Geometry check sheet. Reference: the model listing, model coordinates, mm. Give positions to 0.01 mm unless a question says otherwise; leave off trailing zeros. Loops run counter-clockwise (first coordinate to the right, second up) from the corner with the lowest first, then second, coordinate; pieces in that order, holes last.
1. Material ranges on L1, parallel to Z at x = -4, y = 5; L2, parallel to Z at x = -6, y = 1.5; L3, parallel to Z at x = 9.5, y = 14.5, recorded low to high.
2. Cross-section at A-A, the plane z = -73. Record the cut outline in (x, y), plus the area to 3 significant figures.
3. Cross-section at B-B, the plane y = 12. State how many separate pieces and enclosed holes the cut face has, plus the area to 3 significant figures.
4. Cross-section at C-C, the plane z = -225. Record the cut outline in (x, y).
5. Go/stop test with flat-tipped pins: pin 1 Ø7.5 at (y, z) = (8, -90) entering from +X; pin 2 Ø23.5 at (x, z) = (0, -250) entering from +Y; pin 3 Ø6.5 at (y, z) = (8, -199) entering from -X; pin 4 Ø5 at (x, y) = (-2.5, 3) entering from -Z. Record where each tip stops, or that it passes through.
from build123d import *

# Parameters (mm, degrees)
SKETCH_1_R          = 5.05
SKETCH_1_R_2        = 13
EXTRUDE_1_DEPTH     = 15
FILLET_1_R          = 3
SKETCH_7_R          = 2.05
CUT_EXTRUDE_4_DEPTH = 277.54113618
SKETCH_8_R          = 13
CUT_EXTRUDE_5_DEPTH = 277.54113618
SKETCH_9_R          = 25
SKETCH_9_R_2        = 13
EXTRUDE_4_DEPTH     = 15
SKETCH_10_R         = 1.5
EXTRUDE_5_DEPTH     = 15
EXTRUDE_START       = -15
SKETCH_14_R         = 13
SKETCH_14_R_2       = 9
EXTRUDE_6_DEPTH     = 15
SKETCH_13_R         = 23.5
SKETCH_13_R_2       = 1.5
CUT_EXTRUDE_6_DEPTH = 25
CUT_EXTRUDE_START   = -15
CUT_EXTRUDE_7_DEPTH = 15
EXTRUDE_9_DEPTH     = 15
CUT_EXTRUDE_8_DEPTH = 30


# Read off the part's stored shape, not the designer's step: 切除-拉伸7
with BuildPart() as part:
    # 草图1 → 凸台-拉伸1 (new body)
    with BuildSketch(Plane(origin=(0, 0, 0), x_dir=(1, 0, 0), z_dir=(0, 1, 0))):
        with BuildLine():
            Line((-17.992942616, -0.504), (-24.990198078, 249.3))
            ThreePointArc((-24.990198078, 249.3), (0, 275), (24.990198078, 249.3))
            Line((24.990198078, 249.3), (17.992942616, -0.504))
            ThreePointArc((17.992942616, -0.504), (0, -18), (-17.992942616, -0.504))
        make_face()
        with Locations(Location((0, 0, 0), (0, 0, 270))):
            Circle(SKETCH_1_R, mode=Mode.SUBTRACT)
        with Locations(Location((0, 250, 0), (0, 0, 270))):
            Circle(SKETCH_1_R_2, mode=Mode.SUBTRACT)
        Polygon((-16.444447487, 158.5), (-17.704941698, 203.5), (11.028871219, 137.174942267), align=None, mode=Mode.SUBTRACT)
        Polygon((15.954255294, 141), (18.475243716, 231), (-12, 219.5), align=None, mode=Mode.SUBTRACT)
    extrude(amount=EXTRUDE_1_DEPTH)

    # 圆角1
    fillet_1_edges = [part.edges().sort_by_distance(p)[0] for p in [
        (-16.444447487, 7.5, -158.5),
        (11.028871219, 7.5, -137.174942267),
        (-17.704941698, 7.5, -203.5),
        (18.475243716, 7.5, -231),
        (-12, 7.5, -219.5),
        (15.954255294, 7.5, -141),
    ]]
    fillet(fillet_1_edges, radius=FILLET_1_R)

    # 草图7 → 切除-拉伸4 (cut, through all)
    with BuildSketch(Plane(origin=(0, 15, 0), x_dir=(1, 0, 0), z_dir=(0, 1, 0))):
        with Locations(Location((15, 15, 0), (0, 0, 270))):
            Circle(SKETCH_7_R)
        with Locations(Location((-15, 15, 0), (0, 0, 270))):
            Circle(SKETCH_7_R)
        with Locations((-15, -15)):
            Circle(SKETCH_7_R)
        with Locations((15, -15)):
            Circle(SKETCH_7_R)
    extrude(amount=-CUT_EXTRUDE_4_DEPTH, mode=Mode.SUBTRACT)

    # 草图8 → 切除-拉伸5 (cut, through all)
    with BuildSketch(Plane(origin=(0, 15, 0), x_dir=(1, 0, 0), z_dir=(0, 1, 0))):
        with Locations(Location((0, 0, 0), (0, 0, 270))):
            Circle(SKETCH_8_R)
    extrude(amount=-CUT_EXTRUDE_5_DEPTH, mode=Mode.SUBTRACT)

    # 草图9 → 凸台-拉伸4 (add)
    with BuildSketch(Plane(origin=(0, 15, 0), x_dir=(1, 0, 0), z_dir=(0, 1, 0))):
        Circle(SKETCH_9_R)
        with Locations(Location((0, 0, 0), (0, 0, 270))):
            Circle(SKETCH_9_R_2, mode=Mode.SUBTRACT)
    extrude(amount=-EXTRUDE_4_DEPTH)

    # 草图10 → 凸台-拉伸5 (add)
    with BuildSketch(Plane(origin=(0, 15, 0), x_dir=(1, 0, 0), z_dir=(0, 1, 0))):
        with BuildLine():
            Line((-39.711049207, 4.799226071), (-40, 0))
            ThreePointArc((-40, 0), (0, -40), (40, 0))
            Line((40, 0), (39.711049207, 4.799226071))
            Line((39.711049207, 4.799226071), (24.990198078, 249.3))
            Line((24.990198078, 249.3), (18.993134598, 35.203136766))
            Line((18.993134598, 35.203136766), (18.478724461, 16.838549294))
            ThreePointArc((18.478724461, 16.838549294), (0, -25), (-18.478724461, 16.838549294))
            Line((-18.478724461, 16.838549294), (-18.993134598, 35.203136766))
            Line((-18.993134598, 35.203136766), (-24.990198078, 249.3))
            Line((-24.990198078, 249.3), (-39.711049207, 4.799226071))
        make_face()
        with Locations(Location((-31.493406412, -20.357194124, 0), (0, 0, 270))):
            Circle(SKETCH_10_R, mode=Mode.SUBTRACT)
        with Locations(Location((-37.210701127, 4.649055992, 0), (0, 0, 270))):
            Circle(SKETCH_10_R, mode=Mode.SUBTRACT)
        with Locations(Location((-25.516695234, 27.479961141, 0), (0, 0, 270))):
            Circle(SKETCH_10_R, mode=Mode.SUBTRACT)
        with Locations(Location((-11.039996826, -35.838086864, 0), (0, 0, 270))):
            Circle(SKETCH_10_R, mode=Mode.SUBTRACT)
        with Locations(Location((14.579149971, -34.549940465, 0), (0, 0, 270))):
            Circle(SKETCH_10_R, mode=Mode.SUBTRACT)
        with Locations(Location((33.376550467, -17.095492942, 0), (0, 0, 270))):
            Circle(SKETCH_10_R, mode=Mode.SUBTRACT)
        with Locations(Location((22.631551157, 29.900884473, 0), (0, 0, 270))):
            Circle(SKETCH_10_R, mode=Mode.SUBTRACT)
        with Locations(Location((36.55669206, 8.358125723, 0), (0, 0, 270))):
            Circle(SKETCH_10_R, mode=Mode.SUBTRACT)
    extrude(amount=-EXTRUDE_5_DEPTH)

    # 草图14 → 凸台-拉伸6 (add)
    with BuildSketch(Plane(origin=(0, 15, 0), x_dir=(1, 0, 0), z_dir=(0, 1, 0)).offset(EXTRUDE_START)):
        with Locations((0, 250)):
            Circle(SKETCH_14_R)
        with Locations(Location((0, 250, 0), (0, 0, 270))):
            Circle(SKETCH_14_R_2, mode=Mode.SUBTRACT)
    extrude(amount=EXTRUDE_6_DEPTH)

    # 草图13 → 切除-拉伸6 (cut)
    with BuildSketch(Plane(origin=(0, 15, 0), x_dir=(1, 0, 0), z_dir=(0, 1, 0))):
        with Locations(Location((0, 0, 0), (0, 0, 270))):
            Circle(SKETCH_13_R)
        with Locations(Location((-1.883144055, 37.452687066, 0), (0, 0, 270))):
            Circle(SKETCH_13_R_2)
    extrude(amount=-CUT_EXTRUDE_6_DEPTH, mode=Mode.SUBTRACT)

    # 切除-拉伸7 outline → 切除-拉伸7 (cut)
    with BuildSketch(Plane(origin=(0, 15, 0), x_dir=(1, 0, 0), z_dir=(0, 1, 0)).offset(CUT_EXTRUDE_START)):
        with BuildLine():
            ThreePointArc((-39.711049207, 4.799226071), (-38.432072473, 11.089445679), (-36.163406358, 17.094093734))
            ThreePointArc((-36.163406358, 17.094093734), (-31.834646693, 28.891099747), (-29.684840552, 41.271965817))
            Line((-29.684840552, 41.271965817), (-18, 250))
            ThreePointArc((-18, 250), (0, 268), (18, 250))
            Line((18, 250), (29.684856444, 41.271998774))
            ThreePointArc((29.684856444, 41.271998774), (31.834654407, 28.891107358), (36.163414547, 17.09407641))
            ThreePointArc((36.163414547, 17.09407641), (38.432075129, 11.089436474), (39.711049207, 4.799226071))
            Line((39.711049207, 4.799226071), (24.990198078, 249.3))
            ThreePointArc((24.990198078, 249.3), (0, 275), (-24.990198078, 249.3))
            Line((-24.990198078, 249.3), (-39.711049207, 4.799226071))
        make_face()
    extrude(amount=CUT_EXTRUDE_7_DEPTH, mode=Mode.SUBTRACT)

    # 草图18 → 凸台-拉伸9 (add)
    with BuildSketch(Plane(origin=(0, 0, 0), x_dir=(-1, 0, 0), z_dir=(0, -1, 0))):
        Polygon((-20.868155543, 131.844626328), (20.706902291, 152.097209515), (16.905995412, 230.591726078), (-18.51031166, 232.603381148), (-19.336560971, 196.02914685), align=None)
    extrude(amount=-EXTRUDE_9_DEPTH)

    # 草图19 → 切除-拉伸8 (cut)
    with BuildSketch(Plane(origin=(0, 15, 0), x_dir=(1, 0, 0), z_dir=(0, 1, 0))):
        with BuildLine():
            Line((-7.714285714, 206.181987904), (-7.714285714, 197.835106113))
            ThreePointArc((-7.714285714, 197.835106113), (-7.063735021, 195.368876049), (-5.281369423, 193.544409057))
            Line((-5.281369423, 193.544409057), (1.432916291, 189.52731504))
            ThreePointArc((1.432916291, 189.52731504), (6.466230064, 189.468562789), (9, 193.818012096))
            Line((9, 193.818012096), (9, 202.164893887))
            ThreePointArc((9, 202.164893887), (8.349449307, 204.631123951), (6.567083709, 206.455590943))
            Line((6.567083709, 206.455590943), (-0.147202005, 210.47268496))
            ThreePointArc((-0.147202005, 210.47268496), (-5.180515778, 210.531437211), (-7.714285714, 206.181987904))
        make_face()
        with BuildLine():
            Line((-13, 160.211585543), (-13, 141.864703752))
            ThreePointArc((-13, 141.864703752), (-12.349449307, 139.398473689), (-10.567083709, 137.574006696))
            Line((-10.567083709, 137.574006696), (5.432916291, 128.001357123))
            ThreePointArc((5.432916291, 128.001357123), (10.466230064, 127.942604873), (13, 132.29205418))
            Line((13, 132.29205418), (13, 150.63893597))
            ThreePointArc((13, 150.63893597), (12.349449307, 153.105166034), (10.567083709, 154.929633027))
            Line((10.567083709, 154.929633027), (-5.432916291, 164.5022826))
            ThreePointArc((-5.432916291, 164.5022826), (-10.466230064, 164.56103485), (-13, 160.211585543))
        make_face()
        with BuildLine():
            Line((-15, 100.278326449), (-15, 66.931444658))
            ThreePointArc((-15, 66.931444658), (-14.349449307, 64.465214594), (-12.567083709, 62.640747602))
            Line((-12.567083709, 62.640747602), (7.432916291, 50.674935636))
            ThreePointArc((7.432916291, 50.674935636), (12.466230064, 50.616183385), (15, 54.965632692))
            Line((15, 54.965632692), (15, 88.312514483))
            ThreePointArc((15, 88.312514483), (14.349449307, 90.778744547), (12.567083709, 92.60321154))
            Line((12.567083709, 92.60321154), (-7.432916291, 104.569023505))
            ThreePointArc((-7.432916291, 104.569023505), (-12.466230064, 104.627775756), (-15, 100.278326449))
        make_face()
    extrude(amount=-CUT_EXTRUDE_8_DEPTH, mode=Mode.SUBTRACT)


solid = part.part
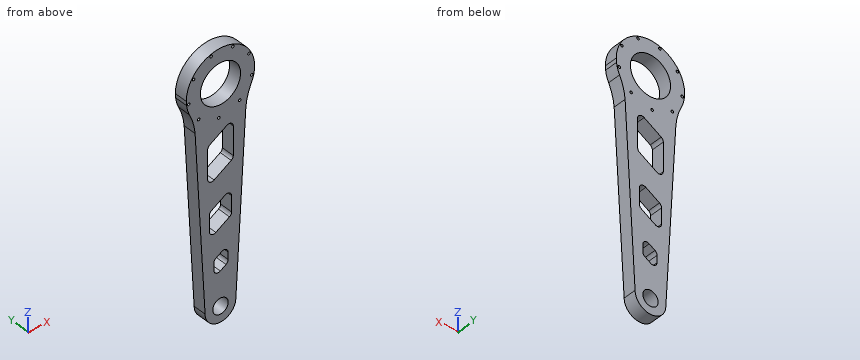
Result:
1. L1: z = -267.55 to -258.06, -241.94 to -211.01, -192.78 to -163.64, -133.64 to -102.52, -57.52 to -23.16, 23.16 to 39.8
1. L2: z = -266.97 to -256.71, -243.29 to -209.95, -194.07 to -164.79, -134.84 to -103.71, -58.71 to -22.72, 22.72 to 39.55
1. L3: z = -265.29 to -155.57, -127.52 to -94.44, -49.99 to -21.49, 21.49 to 38.86
2. outline: (-27.91, 0) - (-15, 0) - (-15, 15) - (-27.91, 15) - close; (15, 0) - (27.91, 0) - (27.91, 15) - (15, 15) - close
2. area: 387 mm2
3. separate pieces: 1
3. enclosed holes: 14
3. area: 11,500 mm2
4. outline: (-19.4, 0) - (19.4, 0) - (19.4, 15) - (-19.4, 15) - close
5. pin 1: stops at x = 27.17
5. pin 2: stops at y = 15
5. pin 3: stops at x = -21.04
5. pin 4: stops at z = -268
